Autodesk Inventor part; units mm, degrees
ref_plane "YZ Plane" through (0, 0, 0) normal (1, 0, 0) x (0, 1, 0)
ref_plane "XZ Plane" through (0, 0, 0) normal (0, 1, 0) x (-1, 0, 0)
ref_plane "XY Plane" through (0, 0, 0) normal (0, 0, 1) x (1, 0, 0)
sketch "Sketch1" plane through (0, 0, 0) normal (0, 1, 0) x (-1, 0, 0)
  line L0 (-10, 24) -> (10, 24)
  line L1 (10, 24) -> (10, -24)
  line L2 (10, -24) -> (-10, -24)
  line L3 (-10, -24) -> (-10, 24)
  line L4 (-10, 24) -> (10, -24) construction
  line L5 (10, 24) -> (-10, -24) construction
  line L6 (0, 0) -> (0, -23.5) construction
  line L7 (0, -23.5) -> (0, -14) construction
  circle A0 centre (0, -14) radius 9.5
  line L8 (0, 0) -> (0, 23.5) construction
  line L9 (0, 23.5) -> (0, 14) construction
  circle A1 centre (0, 14) radius 9.5
  dimension "d0" = 20
  dimension "d1" = 48
  dimension "d2" = 23.5
  dimension "d3" = 9.5
  dimension "d4" = 19
  dimension "d5" = 23.5
  dimension "d6" = 9.5
  dimension "d7" = 19
extrude "Extrusion1" add sketch "Sketch1" along normal blind 25 contours A0 | A1
extrude "Extrusion2" add sketch "Sketch1" against normal blind 10
extrude "Extrusion3" add sketch "Sketch1" against normal blind 10 contours A1
extrude "Extrusion4" add sketch "Sketch1" against normal blind 10 contours A0
properties part number "LIDARLite" material "Acetal Resin, Black"
Source: CAD feature listing. Evaluate the final solid. Frame: model axes, mm. A direction names the side the tool comes from. Round coordinates to 2 decimals unless told otherwise and drop trailing zeros. Order: outer loops, then holes, each group sorted by start corner. A loop starts at its lowest first (then second) coordinate and runs counter-clockwise, first axis right, second up. Notation, with made-up numbers: (10.5, -27) -> (35.5, -27) arc R21 cw to (35.5, -9) -> close; hole circle Ø9 at (-30.75, -6). An arc over 180 degrees is marked (long way). One line per item, written item: value. Start each with the question number.
Q1. Pin query (flat end, axial travel): pin 1 (6 mm diameter, centred on y = 9, z = 1, fed in from +X); pin 2 (3 mm diameter, centred on x = 5.5, y = 20.5, fed in from +Z); pin 3 (12 mm diameter, centred on y = 9.5, z = -16.5, fed in from -X). Return the tip coordinate at first contact, or that it passes through.
Q2. Access query for faces 4 (the flat face through (0, 0, 0)), 5 (the flat face through (10, -5, 0)). Directions: +Z, -Z, +X, -X, +Y, -Y. A direction counts if a zero-diameter tool reaches every point of the face in a straight line with its end or side. Return the directions, or none.
Q3. Section query B-B (z = 14). Return the cut outline in (x, y), plus the area to 3 significant figures.
Q4. Section query A-A (y = 12.5). Return the cut outline in (x, z), plus the area to 3 significant figures.
Q5. Section query C-C (x = 0). Return the cut outline in (y, z).
Q6. Draft query along Z for faces 1 (the flat face through (0, -5, 24)), 2 (the cylindrical face through (-9.061, 12.325, 11.146)), 3 (the flat face through (0, 25, -14)). Return one class per face: pulls with the +Z half, pulls with the -Z half, needs draft (parallel to the pull), parting line crosses it, or undercut.
Q7. Section query D-D (z = -17.5). Return the cut outline in (x, y), plus the area to 3 significant figures.
Q8. Material intervals for probe 1 along Y at (x, z) = (-7, -3); probe 2 along Z at (x, y) = (6, 12); probe 3 along Z at (x, y) = (-4.25, 3), sorted ascending.
Findings below:
1. pin 1: through
1. pin 2: z = 22.62
1. pin 3: x = -9.5
2. face 4: +Y
2. face 5: +Z, -Z, +X, +Y, -Y
3. outline: (-10, -10) -> (10, -10) -> (10, 0) -> (9.5, 0) -> (9.5, 25) -> (-9.5, 25) -> (-9.5, 0) -> (-10, 0) -> close
3. area: 675 mm²
4. outline: circle Ø19 at (0, -14); circle Ø19 at (0, 14)
4. area: 567 mm²
5. outline: (-10, -24) -> (0, -24) -> (0, -23.5) -> (25, -23.5) -> (25, -4.5) -> (0, -4.5) -> (0, 4.5) -> (25, 4.5) -> (25, 23.5) -> (0, 23.5) -> (0, 24) -> (-10, 24) -> close
6. face 1: pulls with the +Z half
6. face 2: undercut
6. face 3: needs draft
7. outline: (-10, -10) -> (10, -10) -> (10, 0) -> (8.83, 0) -> (8.83, 25) -> (-8.83, 25) -> (-8.83, 0) -> (-10, 0) -> close
7. area: 642 mm²
8. probe 1: -10 to 0
8. probe 2: -21.37 to -6.63, 6.63 to 21.37
8. probe 3: -22.5 to -5.5, 5.5 to 22.5
